Design review of the part built by this model. Coordinates are the model's own, in mm. Round coordinates to 2 decimals unless told otherwise and drop trailing zeros. Write each loop counter-clockwise with the first axis right and the second up, starting at its lowest first coordinate (ties: lowest second). Pieces come first, ordered by that corner, then holes. Notation, with made-up numbers: (31.25, 86) - (88.25, 86) arc R21 cw to (88.25, 97) - close; hole circle Ø2 at (-3, -36.75). An arc over 180 degrees is marked (long way). Use one line per item in the form item = value.
Autodesk Inventor part; units mm, degrees
ref_plane "YZ Plane" through (0, 0, 0) normal (1, 0, 0) x (0, 1, 0)
ref_plane "XZ Plane" through (0, 0, 0) normal (0, 1, 0) x (-1, 0, 0)
ref_plane "XY Plane" through (0, 0, 0) normal (0, 0, 1) x (1, 0, 0)
sketch "Sketch1" plane through (0, 0, 0) normal (0, 0, 1) x (1, 0, 0)
  arc A0 (9.652, -11.176) -> (11.176, -9.652) centre (9.652, -9.652) ccw
  line L0 (-9.652, -11.176) -> (9.652, -11.176)
  arc A1 (-11.176, -9.652) -> (-9.652, -11.176) centre (-9.652, -9.652) ccw
  line L1 (-11.176, 9.652) -> (-11.176, -9.652)
  arc A2 (-9.652, 11.176) -> (-11.176, 9.652) centre (-9.652, 9.652) ccw
  line L2 (9.652, 11.176) -> (-9.652, 11.176)
  arc A3 (11.176, 9.652) -> (9.652, 11.176) centre (9.652, 9.652) ccw
  line L3 (11.176, -9.652) -> (11.176, 9.652)
  arc A4 (-12.7, -7.112) -> (-13.462, -6.35) centre (-13.462, -7.112) ccw
  line L4 (-12.7, -7.112) -> (-12.7, -10.5918)
  arc A5 (-12.7, -10.5918) -> (-10.5918, -12.7) centre (-10.5918, -10.5918) ccw
  line L5 (-10.5918, -12.7) -> (10.5918, -12.7)
  arc A6 (10.5918, -12.7) -> (12.7, -10.5918) centre (10.5918, -10.5918) ccw
  line L6 (12.7, -10.5918) -> (12.7, 10.5918)
  arc A7 (12.7, 10.5918) -> (10.5918, 12.7) centre (10.5918, 10.5918) ccw
  line L7 (10.5918, 12.7) -> (-10.5918, 12.7)
  arc A8 (-10.5918, 12.7) -> (-12.7, 10.5918) centre (-10.5918, 10.5918) ccw
  line L8 (-12.7, 10.5918) -> (-12.7, -4.064)
  arc A9 (-13.462, -4.826) -> (-12.7, -4.064) centre (-13.462, -4.064) ccw
  line L9 (-13.462, -4.826) -> (-24.638, -4.826)
  arc A10 (-24.638, -4.826) -> (-24.638, -6.35) centre (-24.638, -5.588) ccw
  line L10 (-24.638, -6.35) -> (-13.462, -6.35)
  point P0 (0, 0)
extrude "Extrusion1" add sketch "Sketch1" against normal blind 304.8
properties part number "9005"
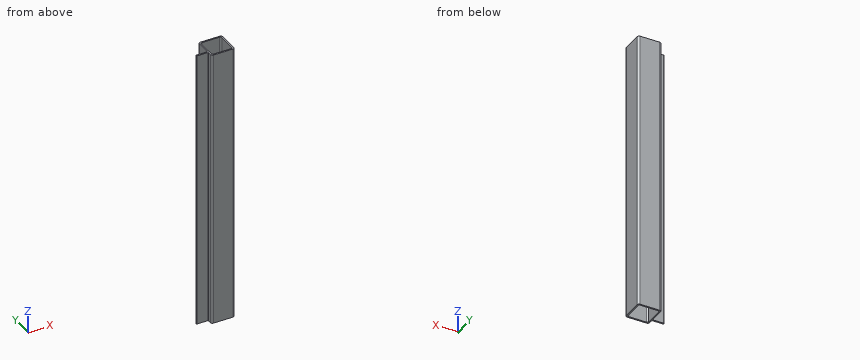
Q1. To check wall thickness, follow line 1 along Y through (x, z) = (8, -217.5); line 2 along Y through (x, z) = (-22.5, -49). State the ranges of each line that lie inside material, in increasing order. Write a range as from..to.
Calculated:
line_1 = -12.7..-11.18, 11.18..12.7
line_2 = -6.35..-4.83
Q2. We need section D-D on x = -21.5. Write out the cut boundary in (y, z).
Calculated:
outline = (-6.35, -304.8) - (-4.83, -304.8) - (-4.83, 0) - (-6.35, 0) - close
Q3. For P1, Ø3, axis at x = -15.5, z = -159.5, coming from the -Y side; P2, Ø3, axis at y = 5.5, z = -226, coming from the -X side; P3, Ø5.5, axis at x = -21.5, z = -187.5, coming from the +Y side, all flat-tipped, find the tip position at first contact; note any pin that passes through.
Calculated:
P1 = -6.35
P2 = -12.7
P3 = -4.83
Q4. We need section A-A on y = 0. Write out the cut boundary in (x, z), then the cut area to 3 significant figures.
Calculated:
outline = (-12.7, -304.8) - (-11.18, -304.8) - (-11.18, 0) - (-12.7, 0) - close; (11.18, -304.8) - (12.7, -304.8) - (12.7, 0) - (11.18, 0) - close
area = 929 mm2
Q5. We need section C-C on z = -257. Write out the cut boundary in (x, y), then the cut area to 3 significant figures.
Calculated:
outline = (-24.64, -6.35) - (-13.46, -6.35) arc R0.76 cw to (-12.7, -7.11) - (-12.7, -10.59) arc R2.11 ccw to (-10.59, -12.7) - (10.59, -12.7) arc R2.11 ccw to (12.7, -10.59) - (12.7, 10.59) arc R2.11 ccw to (10.59, 12.7) - (-10.59, 12.7) arc R2.11 ccw to (-12.7, 10.59) - (-12.7, -4.06) arc R0.76 cw to (-13.46, -4.83) - (-24.64, -4.83) arc R0.76 ccw to start; hole (-11.18, -9.65) arc R1.52 ccw to (-9.65, -11.18) - (9.65, -11.18) arc R1.52 ccw to (11.18, -9.65) - (11.18, 9.65) arc R1.52 ccw to (9.65, 11.18) - (-9.65, 11.18) arc R1.52 ccw to (-11.18, 9.65) - close
area = 163 mm2
